from build123d import *

# Parameters (mm, degrees)
EXTRUDE_1_DEPTH = 15


with BuildPart() as part:
    # Эскиз1 → Бобышка-Вытянуть1 (new body)
    with BuildSketch(Plane(origin=(0, 0, 0), x_dir=(1, 0, 0), z_dir=(0, 1, 0))):
        with BuildLine():
            Line((10, 0), (50, 0))
            ThreePointArc((50, 0), (57.071067812, 2.928932188), (60, 10))
            Line((60, 10), (60, 120))
            Line((60, 120), (0, 120))
            Line((0, 120), (0, 10))
            ThreePointArc((0, 10), (2.928932188, 2.928932188), (10, 0))
        make_face()
        with BuildLine():
            Line((14, 111), (46, 111))
            ThreePointArc((46, 111), (52, 105), (46, 99))
            Line((46, 99), (14, 99))
            ThreePointArc((14, 99), (8, 105), (14, 111))
        make_face(mode=Mode.SUBTRACT)
        with BuildLine():
            Line((14, 91), (46, 91))
            ThreePointArc((46, 91), (52, 85), (46, 79))
            Line((46, 79), (14, 79))
            ThreePointArc((14, 79), (8, 85), (14, 91))
        make_face(mode=Mode.SUBTRACT)
        with BuildLine():
            Line((14, 71), (46, 71))
            ThreePointArc((46, 71), (52, 65), (46, 59))
            Line((46, 59), (14, 59))
            ThreePointArc((14, 59), (8, 65), (14, 71))
        make_face(mode=Mode.SUBTRACT)
        with BuildLine():
            Line((14, 51), (46, 51))
            ThreePointArc((46, 51), (52, 45), (46, 39))
            Line((46, 39), (14, 39))
            ThreePointArc((14, 39), (8, 45), (14, 51))
        make_face(mode=Mode.SUBTRACT)
        with BuildLine():
            Line((14, 31), (46, 31))
            ThreePointArc((46, 31), (52, 25), (46, 19))
            Line((46, 19), (14, 19))
            ThreePointArc((14, 19), (8, 25), (14, 31))
        make_face(mode=Mode.SUBTRACT)
    extrude(amount=EXTRUDE_1_DEPTH)


solid = part.part
Input: part model. Units: mm. Frame: model coordinates. A direction names the side the tool comes from. Give positions to 0.01 mm unless a question says otherwise; leave off trailing zeros. Order: outer loops, then holes, each group sorted by start corner. A loop starts at its lowest first (then second) coordinate and runs counter-clockwise, first axis right, second up.
Q1. Section B-B on y = 7.75. Output: boundary loops of the cut face in (x, z), and give its area (3 significant figures).
Checked values:
outline: (0, -120) - (60, -120) - (60, -10) arc R10 ccw to (50, 0) - (10, 0) arc R10 ccw to (0, -10) - close; hole (14, -111) - (46, -111) arc R6 ccw to (46, -99) - (14, -99) arc R6 ccw to start; hole (14, -91) - (46, -91) arc R6 ccw to (46, -79) - (14, -79) arc R6 ccw to start; hole (14, -71) - (46, -71) arc R6 ccw to (46, -59) - (14, -59) arc R6 ccw to start; hole (14, -51) - (46, -51) arc R6 ccw to (46, -39) - (14, -39) arc R6 ccw to start; hole (14, -31) - (46, -31) arc R6 ccw to (46, -19) - (14, -19) arc R6 ccw to start
area: 4,670 mm2
Q2. Section A-A on x = 20. Output: boundary loops of the cut face in (y, z).
Checked values:
outline: (0, -120) - (15, -120) - (15, -111) - (0, -111) - close; (0, -99) - (15, -99) - (15, -91) - (0, -91) - close; (0, -79) - (15, -79) - (15, -71) - (0, -71) - close; (0, -59) - (15, -59) - (15, -51) - (0, -51) - close; (0, -39) - (15, -39) - (15, -31) - (0, -31) - close; (0, -19) - (15, -19) - (15, 0) - (0, 0) - close
Q3. Section D-D on z = -49. Output: boundary loops of the cut face in (x, y).
Checked values:
outline: (0, 0) - (9.53, 0) - (9.53, 15) - (0, 15) - close; (50.47, 0) - (60, 0) - (60, 15) - (50.47, 15) - close
Q4. Section C-C on z = -85. Output: boundary loops of the cut face in (x, y).
Checked values:
outline: (0, 0) - (8, 0) - (8, 15) - (0, 15) - close; (52, 0) - (60, 0) - (60, 15) - (52, 15) - close
Q5. Ray query, probe 1 along Z at (x, y) = (41.5, 11.75); probe 2 along X at (y, z) = (5.5, -44.5); probe 3 along Z at (x, y) = (12.5, 1.5). Return the intervals inside material, ascending.
Checked values:
probe 1: z = -120 to -111, -99 to -91, -79 to -71, -59 to -51, -39 to -31, -19 to 0
probe 2: x = 0 to 8.02, 51.98 to 60
probe 3: z = -120 to -110.81, -99.19 to -90.81, -79.19 to -70.81, -59.19 to -50.81, -39.19 to -30.81, -19.19 to 0
Q6. Set-up query: faces 1 (the flat face through (30, 7, -59)), 2 (the cylindrical face through (56.99, 7.4, -2.85)). Return all of +Z, -Z, +X, -X, +Y, -Y with unobstructed straight access to the full face (end or side cutting, diameter ignored); none if empty.
Checked values:
face 1: +Y, -Y
face 2: +Z, +X, +Y, -Y
Q7. Draft query along Z for faces 3 (the cylindrical face through (2.85, 7.4, -3.01)), 4 (the cylindrical face through (52, 7, -25)), 5 (the flat face through (30, 7, -120)). Return one class per face: +Z half, -Z half, draft (parallel to the pull), parting line (faces both ways), or undercut.
Checked values:
face 3: +Z half
face 4: undercut
face 5: -Z half
